```python
from build123d import *

# Parameters (mm, degrees)
EXTRUDE_1_DEPTH = 10


with BuildPart() as part:
    # 草图1 → 凸台-拉伸1 (new body)
    with BuildSketch(Plane(origin=(0, 0, 0), x_dir=(1, 0, 0), z_dir=(0, 1, 0))):
        with BuildLine():
            Line((-45, 0), (-45, -30))
            Line((-45, -30), (-50, -30))
            Line((-50, -30), (-50, 30))
            Line((-50, 30), (-45, 30))
            Line((-45, 30), (-45, 21.794494718))
            ThreePointArc((-45, 21.794494718), (0, 50), (45, 21.794494718))
            Line((45, 21.794494718), (45, 30))
            Line((45, 30), (50, 30))
            Line((50, 30), (50, -30))
            Line((50, -30), (45, -30))
            Line((45, -30), (45, 0))
            ThreePointArc((45, 0), (0, 45), (-45, 0))
        make_face()
    extrude(amount=EXTRUDE_1_DEPTH)


solid = part.part
```
Design review of the part built by this model. Coordinates are the model's own, in mm. A direction names the side the tool comes from. Round coordinates to 2 decimals unless told otherwise and drop trailing zeros. Order: outer loops, then holes, each group sorted by start corner. A loop starts at its lowest first (then second) coordinate and runs counter-clockwise, first axis right, second up. Notation, with made-up numbers: (1.25, 70) - (7.25, 70) arc R36 cw to (7.25, 106) - close; hole circle Ø6 at (-21.5, 0). An arc over 180 degrees is marked (long way). One line per question, with ' | ' between items.
Item 1: Draft analysis for pull direction X (two halves, no side actions). For faces 6 (the face through (0, 0, -46)), 7 (the face through (50, 5, 0)), 8 (the face through (45, 5, -26)), state which applies: +X half, -X half, draft (parallel to the pull), parting line (faces both ways), or undercut.
Checks:
face 6: draft | face 7: +X half | face 8: undercut
Item 2: Take a section at B-B, the plane y = 4.5. Write out the cut boundary in (x, z).
Checks:
outline: (-50, -30) - (-45, -30) - (-45, -21.79) arc R50 ccw to (45, -21.79) - (45, -30) - (50, -30) - (50, 30) - (45, 30) - (45, 0) arc R45 cw to (-45, 0) - (-45, 30) - (-50, 30) - close
Item 3: Wall thickness on line 1 (X direction, y = 0.75, z = 27); line 2 (X direction, y = 4, z = -27.5); line 3 (X direction, y = 7.5, z = -39.5): over which ranges is each line inside the solid? List them lowest first. Write a range as [from, to].
Checks:
line 1: [-50, -45], [45, 50] | line 2: [-50, -45], [-41.76, -35.62], [35.62, 41.76], [45, 50] | line 3: [-30.66, -21.56], [21.56, 30.66]
Item 4: Machinability: for faces 1 (the face through (-48, 5, -30)), 2 (the face through (45, 5, 15)), 3 (the face through (48, 5, 30)), 4 (the face through (47, 5, -30)), 5 (the face through (-50, 5, 0)), which of the approach directions +Z, -Z, +X, -X, +Y, -Y give a long, thin tool a straight path to every point of the face, cutting with its end or side? Answer none if there is none.
Checks:
face 1: -Z, -X, +Y, -Y | face 2: +Z, +Y, -Y | face 3: +Z, +X, -X, +Y, -Y | face 4: -Z, +X, +Y, -Y | face 5: +Z, -Z, -X, +Y, -Y
Item 5: Take a section at D-D, the plane z = -42.5. Write out the cut boundary in (x, y), then the cut area to 3 significant figures.
Checks:
outline: (-26.34, 0) - (-14.79, 0) - (-14.79, 10) - (-26.34, 10) - close; (14.79, 0) - (26.34, 0) - (26.34, 10) - (14.79, 10) - close | area: 231 mm²
Item 6: For P1, Ø1, axis at x = 32.5, y = 2.5, coming from the -Z side; P2, Ø1.5, axis at x = 46.5, y = 3, coming from the -Z side; P3, Ø2, axis at x = -15.5, y = 6, coming from the -Z side, all flat-tipped, find the tip position at first contact; note any pin that passes through.
Checks:
P1: z = -38.42 | P2: z = -30 | P3: z = -47.85
Item 7: Take a section at C-C, the plane x = 0. Write out the cut boundary in (y, z).
Checks:
outline: (0, -50) - (10, -50) - (10, -45) - (0, -45) - close
Item 8: Take a section at A-A, the plane z = 6.5. Write out the cut boundary in (x, y).
Checks:
outline: (-50, 0) - (-45, 0) - (-45, 10) - (-50, 10) - close; (45, 0) - (50, 0) - (50, 10) - (45, 10) - close
